from build123d import *

# Parameters (mm, degrees)
SKETCH1_R           = 15
SKETCH1_R_2         = 2
BOSS_EXTRUDE1_DEPTH = 5
BOSS_EXTRUDE2_DEPTH = 5
SKETCH3_R           = 3
CUT_EXTRUDE1_DEPTH  = 2.5
CHAMFER1_SIZE       = 1


with BuildPart() as part:
    # Sketch1 → Boss-Extrude1 (new body)
    with BuildSketch(Plane.XY):
        Circle(SKETCH1_R)
        with Locations((0, 10)):
            Circle(SKETCH1_R_2, mode=Mode.SUBTRACT)
        with Locations((10, 0)):
            Circle(SKETCH1_R_2, mode=Mode.SUBTRACT)
        with Locations((0, -10)):
            Circle(SKETCH1_R_2, mode=Mode.SUBTRACT)
        with Locations((-10, 0)):
            Circle(SKETCH1_R_2, mode=Mode.SUBTRACT)
    extrude(amount=BOSS_EXTRUDE1_DEPTH)

    # Sketch2 → Boss-Extrude2 (add)
    with BuildSketch(Plane.XY.offset(5)):
        with BuildLine():
            Line((-1.5, 6.25), (1.5, 6.25))
            Line((1.5, 6.25), (1.5, 4.769696007))
            ThreePointArc((1.5, 4.769696007), (0, -5), (-1.5, 4.769696007))
            Line((-1.5, 4.769696007), (-1.5, 6.25))
        make_face()
    extrude(amount=BOSS_EXTRUDE2_DEPTH)

    # Sketch3 → Cut-Extrude1 (cut)
    with BuildSketch(Plane.XY.offset(5)):
        with Locations((0, 10)):
            Circle(SKETCH3_R)
        with Locations((-10, 0)):
            Circle(SKETCH3_R)
        with Locations((10, 0)):
            Circle(SKETCH3_R)
        with Locations((0, -10)):
            Circle(SKETCH3_R)
    extrude(amount=-CUT_EXTRUDE1_DEPTH, mode=Mode.SUBTRACT)

    # Chamfer1
    chamfer1_edges = [part.edges().sort_by_distance(p)[0] for p in [
        (-15, 0, 5),
    ]]
    chamfer(chamfer1_edges, length=CHAMFER1_SIZE)


solid = part.part
The listing builds one solid part. Answer for the finished solid, in the listing's coordinates (mm). A direction names the side the tool comes from. Coordinates: 2 decimals unless noted, no trailing zeros. Write each loop counter-clockwise with the first axis right and the second up, starting at its lowest first coordinate (ties: lowest second). Pieces come first, ordered by that corner, then holes. Notation, with made-up numbers: M 52.5,79 L 84.5,79 A7 ccw 84.5,83 Z; hole C 64,-28 d6. An arc over 180 degrees is marked long. Put each result on its own line as item: value. Start each with the question number.
1. For a pull along Y with two mould halves and no side action, classify faces 4 (the flat face through (0, 6.25, 7)), 5 (the flat face through (-8, -1, 2.5)), 6 (the cylindrical face through (-3, 10, 4)), 7 (the flat face through (1.5, 6, 7)) as pulls with the +Y half, pulls with the -Y half, needs draft (parallel to the pull), parting line crosses it, or undercut.
2. A cutting plane is placed at D-D on z = 7.25. Write down the section's boundary in (x, y).
3. A cutting plane is placed at C-C on z = 1.5. Write down the section's boundary in (x, y), then the cut area to 3 significant figures.
4. A cutting plane is placed at B-B on y = 0. Write down the section's boundary in (x, z).
5. Which of the six approach directions +Z, -Z, +X, -X, +Y, -Y give full straight-line access (tool end or side, diameter ignored) to faces 1 (the flat face through (0, 0, 0)), 2 (the flat face through (12, -1, 2.5)), 3 (the flat face through (-1.5, 5, 7))?
6. Flat-ended cylindrical pins translate along their axes: P1, Ø3.5, axis at x = 10, y = 0, coming from the +Z side; P2, Ø1.2, axis at y = 5.5, z = 7, coming from the -X side; P3, Ø4.5, axis at x = 10, y = 0, coming from the +Z side; P4, Ø5, axis at x = 8.5, y = -1, coming from the +Z side. Find the tip coordinate at first contact, or state that the pin passes through.
7. A cutting plane is placed at A-A on x = 0. Write down the section's boundary in (y, z), then the cut area to 3 significant figures.
8. Consider line 1 (Y direction, x = 0, z = 0.85); line 2 (Y direction, x = 0, z = 3.15); line 3 (X direction, y = 2.75, z = 4). Determine where each line is inside the solid, lowest interval first. Write a range as from..to.
Resolved:
1. face 4: pulls with the +Y half
1. face 5: undercut
1. face 6: undercut
1. face 7: needs draft
2. outline: M -1.5,4.77 A5 ccw long 1.5,4.77 L 1.5,6.25 L -1.5,6.25 Z
3. outline: C 0,0 d30; hole C -10,0 d4; hole C 0,-10 d4; hole C 0,10 d4; hole C 10,0 d4
3. area: 657 mm2
4. outline: M -15,0 L -12,0 L -12,2.5 L -13,2.5 L -13,5 L -14,5 L -15,4 Z; M -8,0 L 8,0 L 8,2.5 L 7,2.5 L 7,5 L 5,5 L 5,10 L -5,10 L -5,5 L -7,5 L -7,2.5 L -8,2.5 Z; M 12,0 L 15,0 L 15,4 L 14,5 L 13,5 L 13,2.5 L 12,2.5 Z
5. face 1: -Z, +X, -X, +Y, -Y
5. face 2: +Z
5. face 3: +Z, -X, +Y
6. P1: passes through
6. P2: stops at x = -1.5
6. P3: stops at z = 2.5
6. P4: stops at z = 5
7. outline: M -15,0 L -12,0 L -12,2.5 L -13,2.5 L -13,5 L -14,5 L -15,4 Z; M -8,0 L 8,0 L 8,2.5 L 7,2.5 L 7,5 L 6.25,5 L 6.25,10 L -5,10 L -5,5 L -7,5 L -7,2.5 L -8,2.5 Z; M 12,0 L 15,0 L 15,4 L 14,5 L 13,5 L 13,2.5 L 12,2.5 Z
7. area: 155 mm2
8. line 1: y = -15..-12, -8..8, 12..15
8. line 2: y = -15..-13, -7..7, 13..15
8. line 3: x = -14.75..-11.2, -8.8..8.8, 11.2..14.75
